Source: CAD feature listing. Evaluate the final solid. Frame: model axes, mm. A direction names the side the tool comes from. Round coordinates to 2 decimals unless told otherwise and drop trailing zeros. Write each loop counter-clockwise with the first axis right and the second up, starting at its lowest first coordinate (ties: lowest second). Pieces come first, ordered by that corner, then holes.
Autodesk Inventor part; units mm, degrees
ref_plane "YZ Plane" through (0, 0, 0) normal (1, 0, 0) x (0, 1, 0)
ref_plane "XZ Plane" through (0, 0, 0) normal (0, 1, 0) x (-1, 0, 0)
ref_plane "XY Plane" through (0, 0, 0) normal (0, 0, 1) x (1, 0, 0)
sketch "Sketch1" plane through (0, 0, 0) normal (0, 1, 0) x (-1, 0, 0)
  circle A0 centre (0, 0) radius 9.125
  circle A1 centre (0, 0) radius 12.5
  dimension "d0" = 18.25
  dimension "d1" = 25
extrude "Extrusion1" add sketch "Sketch1" along normal blind 15
sketch "Sketch2" plane through (0, 15, 0) normal (0, 1, 0) x (1, 0, 0)
  line L0 (-12.5, -12.5) -> (12.5, -12.5)
  line L1 (12.5, -12.5) -> (12.5, 12.5)
  line L2 (12.5, 12.5) -> (-12.5, 12.5)
  line L3 (-12.5, 12.5) -> (-12.5, -12.5)
  point P0 (0, 0)
extrude "Extrusion2" add sketch "Sketch2" along normal blind 25
sketch "Sketch3" plane through (12.5, 15, 12.5) normal (1, 0, 0) x (0, 0, -1)
  circle A0 centre (12.5, 12.5) radius 12.5
  circle A1 centre (12.5, 12.5) radius 9.125
  point P0 (12.5, -15)
  dimension "d6" = 25
  dimension "d7" = 18.25
extrude "Extrusion3" add sketch "Sketch3" along normal blind 53.5
fillet "Fillet1" radius 10 5 edges at (0, 40, -12.5) (-12.5, 40, 0) (0, 40, 12.5) (-12.5, 27.5, 12.5) (-12.5, 27.5, -12.5)
sketch "Sketch4" plane through (0, 40, 0) normal (0, 1, 0) x (1, 0, 0)
  circle A0 centre (43.7484, 32.8534) radius 11.25
  circle A1 centre (43.7484, 32.8534) radius 2.75
  circle A2 centre (28.2484, 17.3534) radius 1.75
  circle A3 centre (28.2484, 48.3534) radius 1.75
  circle A4 centre (59.2484, 48.3534) radius 1.75
  circle A5 centre (59.2484, 17.3534) radius 1.75
  line L0 (-2.5, -2.5) -> (-2.5, 2.5)
  line L1 (-2.5, -2.5) -> (55.5607, -2.5)
  line L2 (66, -2.5) -> (66, 83.8642)
  line L3 (55.5607, 83.8642) -> (-2.5, 83.8642)
  line L4 (-2.5, 83.8642) -> (-2.5, -2.5)
  line L5 (-47.4497, 33) -> (137.0981, 33)
  line L6 (43.6, -25.832) -> (43.6, 75.2549)
  line L7 (55.5607, 83.8642) -> (66, 83.8642)
  line L8 (66, -2.5) -> (47.9455, -2.5)
  line L9 (66, -12.5) -> (66, 12.5)
  point P0 (0, 0)
  dimension "d13" = 22.5
  dimension "d14" = 5.5
  dimension "d15" = 3.5
  dimension "d16" = 15.5
  dimension "d20" = 360
  dimension "d37" = 33
  dimension "d43" = 43.6
  dimension "d44" = 0
extrude "Extrusion4" add sketch "Sketch4" against normal blind 3 contours A0 L5 L2 L8 L1 L6 | A0 L5 L4 L3 L7 L2 | L6 L1 L0 L4 L5 A0
fillet "Fillet2" radius 40 1 edges at (-2.5, 38.5, -83.8642)
fillet "Fillet3" radius 10 1 edges at (66, 38.5, -83.8642)
sketch "Sketch5" plane through (66, 27.5, 0) normal (1, 0, 0) x (0, 0, -1)
  circle A0 centre (0, 0) radius 12.5
  line L0 (0, -12.5) -> (-12.5, -12.5)
  line L1 (0, -12.5) -> (73.8642, -12.5)
  line L2 (83.8642, 9.5) -> (83.8642, 12.5)
  line L3 (73.8642, -12.5) -> (73.8642, 12.5)
  line L4 (73.8642, 12.5) -> (0, 12.5)
  circle A1 centre (0, 0) radius 9.125
  line L5 (73.8642, 12.5) -> (73.8642, 9.5)
  point P0 (0, -27.5)
  dimension "d28" = 0
  dimension "d45" = 18.25
extrude "Extrusion5" add sketch "Sketch5" along normal blind 2
fillet "Fillet5" radius 8 2 edges at (67, 15, -73.8642) (68, 27.5, -73.8642)
sketch "Sketch6" plane through (12.5, 15, 0) normal (1, 0, 0) x (0, 0, -1)
  line L0 (12.5, 15) -> (12.5, 0)
  line L1 (12.5, 0) -> (65.8642, 0)
  line L2 (0, 0) -> (65.8642, 0)
  line L3 (65.8642, 0) -> (65.8642, 22)
  line L4 (44.1034, 22) -> (21.6034, 22)
  line L5 (65.8642, 0) -> (12.5, 0)
  line L6 (12.5, 0) -> (12.5, 22)
  line L7 (12.5, 22) -> (65.8642, 22)
  line L8 (65.8642, 22) -> (65.8642, 0)
  point P0 (0, -15)
  point P1 (12.5, 14.9361)
extrude "Extrusion6" add sketch "Sketch6" along normal blind 2
fillet "Fillet6" radius 8 1 edges at (13.5, 15, -65.8642)
sketch "Sketch7" plane through (0, 0, 0) normal (0, -1, 0) x (1, 0, 0)
  circle A0 centre (0, 0) radius 8.975
extrude "Extrusion7" cut sketch "Sketch7" against normal blind 25
sketch "Sketch8" plane through (0, 37, 0) normal (0, -1, 0) x (1, 0, 0)
  line L0 (-23.3822, -55.3999) -> (103.7661, -55.3999)
  line L1 (103.7661, -55.3999) -> (103.7661, -98.1886)
  line L2 (103.7661, -98.1886) -> (-23.3822, -98.1886)
  line L3 (-23.3822, -98.1886) -> (-23.3822, -55.3999)
  point P0 (0, 0)
extrude "Extrusion8" cut sketch "Sketch8" along normal mid plane 200
fillet "Fillet7" radius 8 3 edges at (-0.8005, 38.5, -55.3999) (13.5, 15, -55.3999) (67, 15, -55.3999)
extrude "Extrusion9" cut sketch "Sketch4" against normal blind 200 contours A2 | A5
sketch "Sketch9" plane through (0, 25, 0) normal (0, -1, 0) x (1, 0, 0)
  circle A0 centre (0, 0) radius 7.5
  dimension "d46" = 15
extrude "Extrusion10" cut sketch "Sketch9" against normal blind 60
properties part number "zmotormount"
1) Section query A-A on y = 32. Return the cut outline in (x, z).
Taken from the geometry:
outline: (-12.3, -2.5) arc R9.8 ccw to (-2.5, -12.3) - (12.5, -12.3) - (12.5, -11.66) - (66, -11.66) - (66, -55.4) - (68, -55.4) - (68, -7.94) - (12.5, -7.94) - (12.5, 7.94) - (68, 7.94) - (68, 11.66) - (12.5, 11.66) - (12.5, 12.3) - (-2.5, 12.3) arc R9.8 ccw to (-12.3, 2.5) - close; (12.5, -55.4) - (14.5, -55.4) - (14.5, -12.5) - (12.5, -12.5) - close; hole circle Ø15 at (0, 0)
2) Material intervals for line 1 (X direction, y = 20, z = -24.5); line 2 (Z direction, x = 51, y = 27); line 3 (X direction, y = 29, z = 0), sorted ascending.
Taken from the geometry:
line 1: x = 12.5 to 14.5, 66 to 68
line 2: z = -12.49 to -9.11, 9.11 to 12.49
line 3: x = -12.5 to -7.5, 7.5 to 12.5
3) Reachability of faces 1 (the face through (-11.923, 7.395, -3.755)), 2 (the face through (67, 15, -23)), 3 (the face through (12.5, 36.5, 9)), 4 (the face through (10, 15, 10)) from +Z, -Z, +X, -X, +Y, -Y: full face, straight path, thin tool, end or side. Return the list, or none.
Taken from the geometry:
face 1: -Y
face 2: +Z, -Z, +X, -Y
face 3: +Z, +X, +Y
face 4: +Z, +X, -Y
4) Section query D-D on x = 28.5. Return the cut outline in (y, z) (3 decimals).
Taken from the geometry:
outline: (37, -55.4) - (40, -55.4) - (40, -50.085) - (37, -50.085) - close; (37, -46.622) - (40, -46.622) - (40, -19.085) - (37, -19.085) - close; (37, -15.622) - (40, -15.622) - (40, 2.5) - (39.747, 2.5) arc R12.5 ccw (long way) to (37, -8.124) - close; hole circle Ø18.25 at (27.5, 0)
5) Contact query for flat-ended pins moving along their axis: P1, Ø6.5, axis at y = 21.5, z = -34, coming from the -X side; P2, Ø6, axis at x = 32.5, y = 21.5, coming from the -Z side; P3, Ø16.5, axis at x = 0, z = 0, coming from the -Y side; P4, Ø5, axis at y = 32, z = 6.5, coming from the +X side. Output: stop coordinate, or through.
Taken from the geometry:
P1: stops at x = 12.5
P2: stops at z = -12.13
P3: stops at y = 25
P4: stops at x = 68
6) Section query B-B on x = 50. Return the cut outline in (y, z) (3 decimals).
Taken from the geometry:
outline: (37, -55.4) - (40, -55.4) - (40, -42.206) - (37, -42.206) - close; (37, -23.5) - (40, -23.5) - (40, 2.5) - (39.747, 2.5) arc R12.5 ccw (long way) to (37, -8.124) - close; hole circle Ø18.25 at (27.5, 0)
7) Section query C-C on z = -25.5. Return the cut outline in (x, y).
Taken from the geometry:
outline: (-2.5, 37) - (12.5, 37) - (12.5, 15) - (14.5, 15) - (14.5, 37) - (35.23, 37) - (35.23, 40) - (-2.5, 40) - close; (52.26, 37) - (66, 37) - (66, 15) - (68, 15) - (68, 40) - (52.26, 40) - close
8) Pull-direction query (Y, two-part tool) for faces 5 (the face through (-2.5, 39, -26)), 6 (the face through (13.514, 17.281, -52.994)), 7 (the face through (4.895, 33.831, -11.737)); classes: released by +Y, released by -Y, zero draft, split by the parting line, or undercut.
Taken from the geometry:
face 5: zero draft
face 6: released by -Y
face 7: undercut
